from build123d import *

# Parameters (mm, degrees)
F0_W     = 43.688
F0_H     = 15.875
F1_DEPTH = 5.588
F2_R     = 5.15874
F3_DEPTH = 4.699
F4_R     = 3.96875
F4_W     = 5.588
F4_H     = 15.875
F5_DEPTH = 4.318
F7_D     = 2.5273
F8_SIZE  = 0.508


with BuildPart() as f1:
    # F0 (on Front) → F1 (new body)
    with BuildSketch(Plane.XZ):
        with Locations((21.844, 7.9375)):
            Rectangle(F0_W, F0_H)
    extrude(amount=F1_DEPTH)

    # F2 (on face) → F3 (join)
    with BuildSketch(Plane.YZ.offset(43.688)):
        with BuildLine():
            Line((-12.7, 0), (-5.588, 0))
            Line((-5.588, 0), (-5.588, 15.875))
            Line((-5.588, 15.875), (0, 15.875))
            Line((0, 15.875), (-14.2438521908, 33.520744286))
            ThreePointArc((-14.2438521908, 33.520744286), (-24.8517052521, 35.0496709663), (-27.1580024701, 24.5832887591))
            Line((-27.1580024701, 24.5832887591), (-12.7, 0))
        make_face()
        with Locations((-20.3708, 28.575)):
            Circle(F2_R, mode=Mode.SUBTRACT)
    extrude(amount=-F3_DEPTH)

    # F4 (on face) → F5 (join)
    with BuildSketch(Plane(origin=(0, 0, 0), x_dir=(0, -1, 0), z_dir=(-1, 0, 0))):
        with BuildLine():
            Line((14.2438521908, 33.520744286), (0, 15.875))
            Line((0, 15.875), (5.588, 15.875))
            Line((5.588, 15.875), (5.588, 0))
            Line((5.588, 0), (12.7, 0))
            Line((12.7, 0), (27.1580024701, 24.5832887591))
            ThreePointArc((27.1580024701, 24.5832887591), (24.8517052521, 35.0496709663), (14.2438521908, 33.520744286))
        make_face()
        with Locations((20.3708, 28.575)):
            Circle(F4_R, mode=Mode.SUBTRACT)
        with Locations((2.794, 7.9375)):
            Rectangle(F4_W, F4_H)
    extrude(amount=-F5_DEPTH)

    # F7 (through all)
    with Locations(Plane.XZ.offset(5.588)):
        with Locations((11.1506, 12.7), (30.2006, 12.7), (30.2006, 3.175), (11.1506, 3.175)):
            Hole(F7_D / 2)

    # F8
    f8_edges = [f1.edges().sort_by_distance(p)[0] for p in [
        (4.318, -16.40205, 28.575),
        (38.989, -25.52954, 28.575),
    ]]
    chamfer(f8_edges, length=F8_SIZE)


solid = f1.part
The model under review builds one solid part; all positions refer to its coordinate system, in mm. A direction names the side the tool comes from. Round coordinates to 2 decimals unless told otherwise and drop trailing zeros. Loops run counter-clockwise (first coordinate to the right, second up) from the corner with the lowest first, then second, coordinate; pieces in that order, holes last. Notation, with made-up numbers: M 35.5,10.25 L 48.5,10.25 A5 ccw 48.5,18.25 Z; hole C -7,-1 d3. An arc over 180 degrees is marked long. Answer as CSV lines item,"result". Start each with the question number.
Item 1: For faces 1 (the face through (21, -3, 15.875)), 2 (the face through (41.62, -15.45, 30.12)), 3 (the face through (11.315, -2.755, 13.953)), list the 3-axis set-ups (+Z, -Z, +X, -X, +Y, -Y) from which the entire face can be reached by the end or side of a thin tool; tool diameter is ignored.
Item 2: Consider section B-B (y = -9). Write out the cut boundary in (x, z), then the cut area to 3 significant figures.
Item 3: Consider section D-D (x = 11). Write out the cut boundary in (y, z) (3 decimals), then the cut area to 3 significant figures.
Item 4: Consider section C-C (z = 12.7). Write out the cut boundary in (x, y), then the cut area to 3 significant figures.
Item 5: Consider section A-A (z = 19.5). Write out the cut boundary in (x, y), then the cut area to 3 significant figures.
Item 6: Insertion check: P1, Ø17.5, axis at x = 23, z = 8.5, coming from the -Y side; P2, Ø5, axis at y = -20, z = 18.5, coming from the -X side; P3, Ø5, axis at x = 9, y = -5.5, coming from the +Z side (3 decimals); P4, Ø2, axis at x = 11.15, z = 12.7, coming from the +Y side. Each pin has a flat end and moves straight along its axis. Give the tip position at first contact, or say it passes through.
Item 7: Mouldability with a two-part tool opening along X and no side actions: class faces 4 (the face through (22, -4, 0)), 5 (the face through (43.688, -11, 18)), 6 (the face through (0, -14, 14)), 7 (the face through (31.463, -2.755, 3.231)) as released by +X, released by -X, zero draft, split by the parting line, or undercut.
Item 8: Wall thickness on line 1 (X direction, y = -19.75, z = 18); line 2 (X direction, y = -18.25, z = 24); line 3 (Y direction, x = 15, z = 7.5): over which ranges is each line inside the solid? List them lowest first. Write a range as [from, to].
Answer:
1,face 1,"+Z, +Y, -Y"
1,face 2,"+X"
1,face 3,"+Y, -Y"
2,outline,"M 0,0 L 4.32,0 L 4.32,27.02 L 0,27.02 Z; M 38.99,0 L 43.69,0 L 43.69,27.02 L 38.99,27.02 Z"
2,area,"244 mm^2"
3,outline,"M -5.588,0 L 0,0 L 0,1.92 L -5.588,1.92 Z; M -5.588,4.43 L 0,4.43 L 0,11.445 L -5.588,11.445 Z; M -5.588,13.955 L 0,13.955 L 0,15.875 L -5.588,15.875 Z"
3,area,"60.7 mm^2"
4,outline,"M 0,-20.17 L 4.32,-20.17 L 4.32,-5.59 L 9.89,-5.59 L 9.89,0 L 0,0 Z; M 12.41,-5.59 L 28.94,-5.59 L 28.94,0 L 12.41,0 Z; M 31.46,-5.59 L 38.99,-5.59 L 38.99,-20.17 L 43.69,-20.17 L 43.69,0 L 31.46,0 Z"
4,area,"347 mm^2"
5,outline,"M 0,-24.17 L 4.32,-24.17 L 4.32,-2.93 L 0,-2.93 Z; M 38.99,-24.17 L 43.69,-24.17 L 43.69,-2.93 L 38.99,-2.93 Z"
5,area,"192 mm^2"
6,P1,"stops at y = -5.59"
6,P2,"stops at x = 0"
6,P3,"stops at z = 15.875"
6,P4,"passes through"
7,face 4,"zero draft"
7,face 5,"released by +X"
7,face 6,"released by -X"
7,face 7,"undercut"
8,line 1,"x = [0, 4.32], [38.99, 43.69]"
8,line 2,"x = [0, 4.32]"
8,line 3,"y = [-5.59, 0]"
